The listing builds one solid part. Answer for the finished solid, in the listing's coordinates (mm). A direction names the side the tool comes from. Coordinates: 2 decimals unless noted, no trailing zeros. Loops run counter-clockwise (first coordinate to the right, second up) from the corner with the lowest first, then second, coordinate; pieces in that order, holes last. Notation, with made-up numbers: (29.5, 87) -> (57.5, 87) arc R18 ccw to (57.5, 111) -> close; hole circle Ø2 at (17, -27). An arc over 180 degrees is marked (long way). Answer in a Markdown table with one row per item.
```python
from build123d import *

# Parameters (mm, degrees)
PAD_DEPTH       = 17.25
SKETCH001_R     = 2.35
POCKET_DEPTH    = 21.001
POCKET001_DEPTH = 3.9
SKETCH003_R     = 4.45
POCKET002_DEPTH = 3
SKETCH004_R     = 1.925
POCKET003_DEPTH = 23.501
POCKET004_DEPTH = 3
SKETCH006_R     = 1.925
POCKET005_DEPTH = 2


with BuildPart() as part:
    # Sketch → Pad (new body, symmetric)
    with BuildSketch(Plane.XZ):
        Polygon((0, 0), (23.5, 0), (23.5, 7), (7, 7), (7, 14), (23.5, 14), (23.5, 21), (0, 21), align=None)
    extrude(amount=PAD_DEPTH, both=True)

    # Sketch001 → Pocket (cut, through all)
    with BuildSketch(Plane(origin=(0, 0, 21), x_dir=(-1, 0, 0), z_dir=(0, 0, 1))):
        with Locations((-15, 8.25)):
            Circle(SKETCH001_R)
        with Locations((-15, -8.25)):
            Circle(SKETCH001_R)
    extrude(amount=-POCKET_DEPTH, mode=Mode.SUBTRACT)

    # Sketch002 → Pocket001 (cut)
    with BuildSketch(Plane(origin=(0, 0, 0), x_dir=(1, 0, 0), z_dir=(0, 0, -1))):
        Polygon((15, 12.75), (11.102886, 10.5), (11.102886, 6), (15, 3.75), (18.897114, 6), (18.897114, 10.5), align=None)
        Polygon((15, -3.75), (11.102886, -6), (11.102886, -10.5), (15, -12.75), (18.897114, -10.5), (18.897114, -6), align=None)
    extrude(amount=-POCKET001_DEPTH, mode=Mode.SUBTRACT)

    # Sketch003 → Pocket002 (cut)
    with BuildSketch(Plane(origin=(0, 0, 21), x_dir=(-1, 0, 0), z_dir=(0, 0, 1))):
        with Locations((-15, 8.25)):
            Circle(SKETCH003_R)
        with Locations((-15, -8.25)):
            Circle(SKETCH003_R)
    extrude(amount=-POCKET002_DEPTH, mode=Mode.SUBTRACT)

    # Sketch004 → Pocket003 (cut, through all)
    with BuildSketch(Plane(origin=(0, 0, 0), x_dir=(0, 0, -1), z_dir=(-1, 0, 0))):
        with Locations((-10.5, 0)):
            Circle(SKETCH004_R)
    extrude(amount=-POCKET003_DEPTH, mode=Mode.SUBTRACT)

    # Sketch005 → Pocket004 (cut)
    with BuildSketch(Plane(origin=(7, 0, 0), x_dir=(0, 0, 1), z_dir=(1, 0, 0))):
        Polygon((7, 2.020726), (7, -2.020726), (10.5, -4.041452), (14, -2.020726), (14, 2.020726), (10.5, 4.041452), align=None)
    extrude(amount=-POCKET004_DEPTH, mode=Mode.SUBTRACT)

    # Sketch006 → Pocket005 (cut)
    with BuildSketch(Plane(origin=(0, 0, 0), x_dir=(0, 0, -1), z_dir=(-1, 0, 0))):
        with Locations((-10.5, -8.5)):
            Circle(SKETCH006_R)
        with Locations((-10.5, 8.5)):
            Circle(SKETCH006_R)
    extrude(amount=-POCKET005_DEPTH, mode=Mode.SUBTRACT)


solid = part.part
```
Item 1: A cutting plane is placed at C-C, the plane z = 2. Determine the outline of the cut face in (x, y).
Findings below:
| item | result |
|---|---|
| outline | (0, -17.25) -> (23.5, -17.25) -> (23.5, 17.25) -> (0, 17.25) -> close; hole (11.1, -10.5) -> (15, -12.75) -> (18.9, -10.5) -> (18.9, -6) -> (15, -3.75) -> (11.1, -6) -> close; hole (11.1, 6) -> (15, 3.75) -> (18.9, 6) -> (18.9, 10.5) -> (15, 12.75) -> (11.1, 10.5) -> close |
Item 2: A cutting plane is placed at D-D, the plane y = 11. Determine the outline of the cut face in (x, z), plus the area to 3 significant figures.
Findings below:
| item | result |
|---|---|
| outline | (0, 0) -> (11.97, 0) -> (11.97, 3.9) -> (18.03, 3.9) -> (18.03, 0) -> (23.5, 0) -> (23.5, 7) -> (7, 7) -> (7, 14) -> (23.5, 14) -> (23.5, 21) -> (18.5, 21) -> (18.5, 18) -> (11.5, 18) -> (11.5, 21) -> (0, 21) -> close |
| area | 333 mm2 |
Item 3: Find the intervals of material crossed by probe 1 along Y at (x, z) = (15, 18.8); probe 2 along Y at (x, z) = (15, 6.4); probe 3 along Y at (x, z) = (1.55, 10.5) (3 decimals), in increasing order.
Findings below:
| item | result |
|---|---|
| probe 1 | y = -17.25 to -12.7, -3.8 to 3.8, 12.7 to 17.25 |
| probe 2 | y = -17.25 to -10.6, -5.9 to 5.9, 10.6 to 17.25 |
| probe 3 | y = -17.25 to -10.425, -6.575 to -1.925, 1.925 to 6.575, 10.425 to 17.25 |
Item 4: A tool of negligible diameter and unlimited length cuts with its end or side. For faces 1 (the face through (19.446, 8.054, 19.521)), 2 (the face through (5.5, 3, 8.7)), 3 (the face through (16.92, -4.86, 1.92)), from which of +Z, -Z, +X, -X, +Y, -Y can it reach the whole face along a straight path? Write none if from no direction.
Findings below:
| item | result |
|---|---|
| face 1 | +Z |
| face 2 | +X |
| face 3 | -Z |
Item 5: A cutting plane is placed at A-A, the plane y = 0. Determine the outline of the cut face in (x, z) (3 decimals).
Findings below:
| item | result |
|---|---|
| outline | (0, 0) -> (23.5, 0) -> (23.5, 7) -> (4, 7) -> (4, 8.575) -> (0, 8.575) -> close; (0, 12.425) -> (4, 12.425) -> (4, 14) -> (23.5, 14) -> (23.5, 21) -> (0, 21) -> close |
Item 6: A cutting plane is placed at B-B, the plane x = 6.25. Determine the outline of the cut face in (y, z), plus the area to 3 significant figures.
Findings below:
| item | result |
|---|---|
| outline | (-17.25, 0) -> (17.25, 0) -> (17.25, 21) -> (-17.25, 21) -> close; hole (-4.04, 10.5) -> (-2.02, 7) -> (2.02, 7) -> (4.04, 10.5) -> (2.02, 14) -> (-2.02, 14) -> close |
| area | 682 mm2 |
Item 7: Determine the mould class of faces 4 (the face through (6, -17.25, 11)), 5 (the face through (17, 10, 3.9)), 6 (the face through (7, 10, 10)) for opening direction X: +X half, -X half, draft (parallel to the pull), parting line (faces both ways), or undercut.
Findings below:
| item | result |
|---|---|
| face 4 | draft |
| face 5 | undercut |
| face 6 | +X half |
Item 8: Flat-ended cylindrical pins translate along their axes: pin 1 Ø2.5 at (y, z) = (8.5, 10.5) entering from -X; pin 2 Ø5 at (y, z) = (-8.5, 10.5) entering from +X; pin 3 Ø5.5 at (x, y) = (15, -8.25) entering from +Z. Find the tip coordinate at first contact, or state that the pin passes through.
Findings below:
| item | result |
|---|---|
| pin 1 | stops at x = 2 |
| pin 2 | stops at x = 7 |
| pin 3 | stops at z = 18 |
